```python
from build123d import *

# Parameters (mm, degrees)
SKETCH_1_R          = 0.6
SKETCH_1_W          = 4.5
SKETCH_1_H          = 10
SKETCH_1_R_2        = 0.65
SKETCH_1_W_2        = 1
SKETCH_1_W_3        = 2.5
SKETCH_1_H_2        = 2
EXTRUDE_1_DEPTH     = 1
EXTRUDE_START       = 1
SKETCH_1_4_W        = 1
SKETCH_1_4_H        = 10
EXTRUDE_2_DEPTH     = 1
SKETCH_2_W          = 1
SKETCH_2_H          = 8
CUT_EXTRUDE_1_DEPTH = 0.5


with BuildPart() as part:
    # 草图1 → 凸台-拉伸1 (new body)
    # profile 1 of 7: a face of its own
    with BuildSketch(Plane(origin=(0, 0, 0), x_dir=(0, 0, -1), z_dir=(1, 0, 0))):
        Polygon((0, 2), (0, 0), (4.5, 0), (5.5, 0), (10, 0), (10, 2), align=None)
        with Locations((1.042294057, 1)):
            Circle(SKETCH_1_R, mode=Mode.SUBTRACT)
        with Locations((4.542294057, 1)):
            Circle(SKETCH_1_R, mode=Mode.SUBTRACT)
    # profile 2 of 7: a face of its own
    with BuildSketch(Plane(origin=(0, 0, 0), x_dir=(0, 0, -1), z_dir=(1, 0, 0))):
        with Locations((2.25, -5)):
            Rectangle(SKETCH_1_W, SKETCH_1_H)
        with Locations((3.2, -9)):
            Circle(SKETCH_1_R_2, mode=Mode.SUBTRACT)
        with Locations((3.2, -1)):
            Circle(SKETCH_1_R_2, mode=Mode.SUBTRACT)
    # profile 3 of 7: a face of its own
    with BuildSketch(Plane(origin=(0, 0, 0), x_dir=(0, 0, -1), z_dir=(1, 0, 0))):
        Polygon((0, -10), (0, 0), (0, 2), (-1, 2), (-1, -10.9), (0, -10.9), align=None)
    # profile 4 of 7: a face of its own
    with BuildSketch(Plane(origin=(0, 0, 0), x_dir=(0, 0, -1), z_dir=(1, 0, 0))):
        with Locations((5, -5)):
            Rectangle(SKETCH_1_W_2, SKETCH_1_H)
    # profile 5 of 7: a face of its own
    with BuildSketch(Plane(origin=(0, 0, 0), x_dir=(0, 0, -1), z_dir=(1, 0, 0))):
        Polygon((4.5, -10), (0, -10), (0, -10.9), (4.05, -10.9), (6.55, -10.9), (10, -10.9), (10, -10), (5.5, -10), align=None)
    # profile 6 of 7: a face of its own
    with BuildSketch(Plane(origin=(0, 0, 0), x_dir=(0, 0, -1), z_dir=(1, 0, 0))):
        with Locations((7.75, -5)):
            Rectangle(SKETCH_1_W, SKETCH_1_H)
        with Locations((6.8, -9)):
            Circle(SKETCH_1_R_2, mode=Mode.SUBTRACT)
        with Locations((6.8, -1)):
            Circle(SKETCH_1_R_2, mode=Mode.SUBTRACT)
    # profile 7 of 7: a face of its own
    with BuildSketch(Plane(origin=(0, 0, 0), x_dir=(0, 0, -1), z_dir=(1, 0, 0))):
        with Locations((5.3, -11.9)):
            Rectangle(SKETCH_1_W_3, SKETCH_1_H_2)
        with Locations((5.3, -11.9)):
            Circle(SKETCH_1_R, mode=Mode.SUBTRACT)
    extrude(amount=EXTRUDE_1_DEPTH)

    # 草图1<4> → 凸台-拉伸2 (add)
    with BuildSketch(Plane(origin=(0, 0, 0), x_dir=(0, 0, -1), z_dir=(1, 0, 0)).offset(EXTRUDE_START)):
        with Locations((5, -5)):
            Rectangle(SKETCH_1_4_W, SKETCH_1_4_H)
    extrude(amount=EXTRUDE_2_DEPTH)

    # 草图2 → 切除-拉伸1 (cut)
    with BuildSketch(Plane(origin=(1, 0, 0), x_dir=(0, 0, -1), z_dir=(1, 0, 0))):
        with Locations((6.8, -5.415331193)):
            Rectangle(SKETCH_2_W, SKETCH_2_H)
        with Locations((3.2, -5.415331193)):
            Rectangle(SKETCH_2_W, SKETCH_2_H)
    extrude(amount=-CUT_EXTRUDE_1_DEPTH, mode=Mode.SUBTRACT)


solid = part.part
```
Work out the finished part from the listing and answer in its coordinate system (mm). A direction names the side the tool comes from. Coordinates: 2 decimals unless noted, no trailing zeros. Loops run counter-clockwise (first coordinate to the right, second up) from the corner with the lowest first, then second, coordinate; pieces in that order, holes last. Notation, with made-up numbers: (15.5, 3.25) - (42.5, 3.25) arc R11 ccw to (42.5, 18.25) - close; hole circle Ø8 at (73.5, 65). An arc over 180 degrees is marked (long way). Use a Markdown table: item, result.
Item 1: Find section D-D, the plane y = 1. Determine the outline of the cut face in (x, z).
Evaluation:
| item | result |
|---|---|
| outline | (0, -10) - (1, -10) - (1, -5.14) - (0, -5.14) - close; (0, -3.94) - (1, -3.94) - (1, -1.64) - (0, -1.64) - close; (0, -0.44) - (1, -0.44) - (1, 1) - (0, 1) - close |
Item 2: Find section A-A, the plane y = -11.9. Determine the outline of the cut face in (x, z), and give its area (3 significant figures).
Evaluation:
| item | result |
|---|---|
| outline | (0, -6.55) - (1, -6.55) - (1, -5.9) - (0, -5.9) - close; (0, -4.7) - (1, -4.7) - (1, -4.05) - (0, -4.05) - close |
| area | 1.30 mm2 |
Item 3: Find section C-C, the plane z = -5.3. Determine the outline of the cut face in (x, y).
Evaluation:
| item | result |
|---|---|
| outline | (0, -12.9) - (1, -12.9) - (1, -12.5) - (0, -12.5) - close; (0, -11.3) - (1, -11.3) - (1, -10) - (2, -10) - (2, 0) - (1, 0) - (1, 2) - (0, 2) - close |
Item 4: Given pin 1 Ø0.5 at (y, z) = (-5.5, -6.5) entering from +X; pin 2 Ø1.1 at (x, z) = (0.5, -8.5) entering from -Y; pin 3 Ø0.8 at (x, y) = (1.5, -3.5) entering from -Z, each flat-ended and moving along its own axis, determine where each tip first touches the part or whether it passes through.
Evaluation:
| item | result |
|---|---|
| pin 1 | stops at x = 1 |
| pin 2 | stops at y = -10.9 |
| pin 3 | stops at z = -5.5 |
Item 5: Consider probe 1 along Z at (x, y) = (0.45, -9); probe 2 along Y at (x, z) = (0.4, -6.8); probe 3 along X at (y, z) = (-3.5, 0). Determine where each line is inside the solid, lowest interval first. Write a range as from..to.
Evaluation:
| item | result |
|---|---|
| probe 1 | z = -10..-7.45, -6.15..-3.85, -2.55..1 |
| probe 2 | y = -10.9..-9.65, -8.35..-1.65, -0.35..2 |
| probe 3 | x = 0..1 |
Item 6: The mould has two halves that part along Z. Classify faces 6 (the cylindrical face through (0.493, -0.356, -6.715)), 7 (the flat face through (0.5, -4.5, -10)), 8 (the flat face through (1, -5, -4)): +Z half, -Z half, draft (parallel to the pull), parting line (faces both ways), or undercut.
Evaluation:
| item | result |
|---|---|
| face 6 | undercut |
| face 7 | -Z half |
| face 8 | draft |
Item 7: For faces 1 (the flat face through (0.5, -10.9, -8.3)), 2 (the flat face through (0.5, -10.9, -1.5)), 3 (the flat face through (0.5, -5, -7)), 4 (the flat face through (1.5, -5.1, -4.5)), 5 (the flat face through (1.5, 0, -5)), determine the directions among +Z, -Z, +X, -X, +Y, -Y from which every point of the face is accessible in a straight line to the end or side of a thin tool.
Evaluation:
| item | result |
|---|---|
| face 1 | -Z, +X, -X, -Y |
| face 2 | +Z, +X, -X, -Y |
| face 3 | +X |
| face 4 | +Z, +X, +Y, -Y |
| face 5 | +Z, -Z, +X, +Y |
Item 8: Find section B-B, the plane z = -3.2. Determine the outline of the cut face in (x, y), and give its area (3 significant figures).
Evaluation:
| item | result |
|---|---|
| outline | (0, -10.9) - (1, -10.9) - (1, -9.65) - (0, -9.65) - close; (0, -8.35) - (0.5, -8.35) - (0.5, -1.65) - (0, -1.65) - close; (0, -0.35) - (1, -0.35) - (1, 2) - (0, 2) - close |
| area | 6.95 mm2 |
